Autodesk Inventor part; units mm, degrees
ref_plane "YZ Plane" through (0, 0, 0) normal (1, 0, 0) x (0, 1, 0)
ref_plane "XZ Plane" through (0, 0, 0) normal (0, 1, 0) x (-1, 0, 0)
ref_plane "XY Plane" through (0, 0, 0) normal (0, 0, 1) x (1, 0, 0)
sketch "Sketch1" plane through (0, 0, 0) normal (0, 0, 1) x (1, 0, 0)
  line L0 (0, 0) -> (25.4, 0)
  line L1 (25.4, 0) -> (25.4, 50.8)
  line L2 (25.4, 50.8) -> (0, 50.8)
  line L3 (0, 50.8) -> (0, 0)
  line L4 (1.5875, 49.2125) -> (23.8125, 49.2125)
  line L5 (23.8125, 49.2125) -> (23.8125, 1.5875)
  line L6 (23.8125, 1.5875) -> (1.5875, 1.5875)
  line L7 (1.5875, 1.5875) -> (1.5875, 49.2125)
  dimension "d0" = 25.4
  dimension "d1" = 50.8
  dimension "d2" = 1.5875
extrude "Extrusion1" add sketch "Sketch1" along normal blind 653.34
sketch "Sketch2" plane through (0, 50.8, 0) normal (0, 1, 0) x (1, 0, 0)
  line L0 (25.4, 0) -> (0, 0) construction
  line L1 (12.7, 0) -> (12.7, -12.7) construction
  line L2 (12.7, -12.7) -> (12.7, -38.1) construction
  line L3 (0, -653.34) -> (25.4, -653.34) construction
  line L4 (12.7, -653.34) -> (12.7, -640.64) construction
  line L5 (12.7, -640.64) -> (12.7, -615.24) construction
  circle A0 centre (12.7, -640.64) radius 2.5797
  circle A1 centre (12.7, -615.24) radius 2.5797
  circle A2 centre (12.7, -38.1) radius 2.5797
  circle A3 centre (12.7, -12.7) radius 2.5797
  dimension "d5" = 12.7
  dimension "d6" = 25.4
  dimension "d7" = 12.7
  dimension "d8" = 25.4
  dimension "d9" = 5.1594
extrude "Extrusion2" cut sketch "Sketch2" against normal blind 653.34
sketch "Sketch3" plane through (25.4, 0, 0) normal (1, 0, 0) x (0, 0, -1)
  line L0 (0, 50.8) -> (-653.34, 50.8) construction
  line L1 (-326.67, 50.8) -> (-326.67, 0) construction
  line L2 (0, 0) -> (-653.34, 0) construction
  line L3 (0, 49.2125) -> (0, 1.5875) construction
  line L4 (0, 25.4) -> (-110.77, 25.4) construction
  circle A0 centre (-110.77, 25.4) radius 7.9375
  circle A1 centre (-542.57, 25.4) radius 7.9375
  dimension "d12" = 110.77
  dimension "d13" = 15.875
extrude "Extrusion3" cut sketch "Sketch3" against normal blind 653.34
properties part number "1x2 piston attachment"
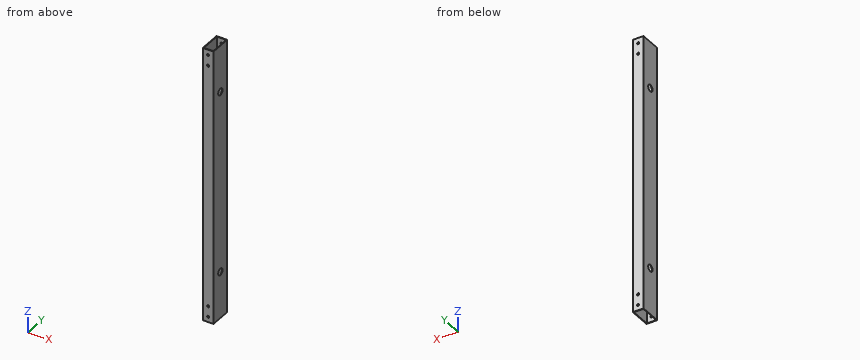
Verification items for the finished model (mm, model axes). Give positions to 0.01 mm unless a question says otherwise; leave off trailing zeros. Loops run counter-clockwise (first coordinate to the right, second up) from the corner with the lowest first, then second, coordinate; pieces in that order, holes last.
1) Sectioned sample at A-A, the plane z = 542.57. Enter the section's corners in (x, y).
2) Sectioned sample at B-B, the plane x = 20. Enter the section's corners in (y, z), then the cut area to 3 significant figures.
3) Sectioned sample at C-C, the plane z = 236. Enter the section's corners in (x, y).
4) Thickness scan on line 1 along Z through (x, y) = (12.7, 49.8); line 2 along X through (y, z) = (30.5, 532.5); line 3 along Y through (x, z) = (21.5, 504). Record the ranges inside material, lowest first.
Answers:
1. outline: (0, 0) - (25.4, 0) - (25.4, 17.46) - (23.81, 17.46) - (23.81, 1.59) - (1.59, 1.59) - (1.59, 17.46) - (0, 17.46) - close; (0, 33.34) - (1.59, 33.34) - (1.59, 49.21) - (23.81, 49.21) - (23.81, 33.34) - (25.4, 33.34) - (25.4, 50.8) - (0, 50.8) - close
2. outline: (0, 0) - (1.59, 0) - (1.59, 653.34) - (0, 653.34) - close; (49.21, 0) - (50.8, 0) - (50.8, 653.34) - (49.21, 653.34) - close
2. area: 2,070 mm2
3. outline: (0, 0) - (25.4, 0) - (25.4, 50.8) - (0, 50.8) - close; hole (1.59, 1.59) - (23.81, 1.59) - (23.81, 49.21) - (1.59, 49.21) - close
4. line 1: z = 0 to 10.12, 15.28 to 35.52, 40.68 to 612.66, 617.82 to 638.06, 643.22 to 653.34
4. line 2: x = 0 to 1.59, 23.81 to 25.4
4. line 3: y = 0 to 1.59, 49.21 to 50.8
